```python
from build123d import *

# Parameters (mm, degrees)
SKETCH_W     = 15
SKETCH_H     = 15
PAD_DEPTH    = 4
SKETCH001_R  = 5.5
POCKET_DEPTH = 2.5


with BuildPart() as part:
    # Sketch → Pad (new body, symmetric)
    with BuildSketch(Plane.XY):
        Rectangle(SKETCH_W, SKETCH_H)
    extrude(amount=PAD_DEPTH, both=True)

    # Sketch001 → Pocket (cut, symmetric)
    with BuildSketch(Plane.XY):
        Circle(SKETCH001_R)
    extrude(amount=POCKET_DEPTH, both=True, mode=Mode.SUBTRACT)


solid = part.part
```
Check sheet for the modelled part. Datum: model origin and axes. Units: mm. A direction names the side the tool comes from. Round coordinates to 2 decimals unless told otherwise and drop trailing zeros. Write each loop counter-clockwise with the first axis right and the second up, starting at its lowest first coordinate (ties: lowest second). Pieces come first, ordered by that corner, then holes. Notation, with made-up numbers: (4.5, 57.5) -> (35.5, 57.5) arc R27 cw to (35.5, 84.5) -> close; hole circle Ø1 at (43.5, 41.25). An arc over 180 degrees is marked (long way). One line per question, with ' | ' between items. Start each with the question number.
1. Sectioned sample at A-A, the plane x = 0. Record the cut outline in (y, z), then the cut area to 3 significant figures.
2. Scan lines: line 1 along Z through (x, y) = (-2.75, 4.5); line 2 along Y through (x, z) = (0, -1.35); line 3 along Y through (x, z) = (-2.75, -2). Record each from-to range of solid material in increasing order. Write a range as from..to.
3. Release check for a two-part mould opening along X. For faces 1 (the face through (0, 0, 4)), 2 (the face through (7.5, 0, 0)), 3 (the face through (0, 0, 2.5)) record: +X half, -X half, draft (parallel to the pull), parting line (faces both ways), or undercut.
4. Set-up check for faces 4 (the face through (-1.19, -5.37, 0.04)), 5 (the face through (0, 7.5, 0)): record each of +Z, -Z, +X, -X, +Y, -Y from which the full face is reachable in a straight line by a thin tool's end or side.
5. Sectioned sample at C-C, the plane z = -2. Record the cut outline in (x, y), then the cut area to 3 significant figures.
Taken from the geometry:
1) outline: (-7.5, -4) -> (7.5, -4) -> (7.5, 4) -> (-7.5, 4) -> close; hole (-5.5, -2.5) -> (5.5, -2.5) -> (5.5, 2.5) -> (-5.5, 2.5) -> close | area: 65.0 mm^2
2) line 1: z = -4..-2.5, 2.5..4 | line 2: y = -7.5..-5.5, 5.5..7.5 | line 3: y = -7.5..-4.76, 4.76..7.5
3) face 1: draft | face 2: +X half | face 3: undercut
4) face 4: none | face 5: +Z, -Z, +X, -X, +Y
5) outline: (-7.5, -7.5) -> (7.5, -7.5) -> (7.5, 7.5) -> (-7.5, 7.5) -> close; hole circle Ø11 at (0, 0) | area: 130 mm^2
